Check sheet for the modelled part. Datum: model origin and axes. Units: mm. Face numbers are marked on the shaded views. A direction names the side the tool comes from. Round coordinates to 2 decimals unless told otherwise and drop trailing zeros. Order: outer loops, then holes, each group sorted by start corner. A loop starts at its lowest first (then second) coordinate and runs counter-clockwise, first axis right, second up.
```python
from build123d import *

# Parameters (mm, degrees)
CROQUIS1_R              = 10
SALIENTE_EXTRUIR1_DEPTH = 3.96875
CROQUIS3_W              = 30
CROQUIS3_H              = 7.9375
SALIENTE_EXTRUIR2_DEPTH = 30
CROQUIS4_R              = 3.175
CORTAR_EXTRUIR1_DEPTH   = 60


with BuildPart() as part:
    # Croquis1 → Saliente-Extruir1 (new, symmetric)
    with BuildSketch(Plane.XY):
        with BuildLine():
            Line((-30, -20), (30, -20))
            Line((30, -20), (30, 0))
            ThreePointArc((30, 0), (24.142135624, 14.142135624), (10, 20))
            Line((10, 20), (-10, 20))
            ThreePointArc((-10, 20), (-24.142135624, 14.142135624), (-30, 0))
            Line((-30, 0), (-30, -20))
        make_face()
        Circle(CROQUIS1_R, mode=Mode.SUBTRACT)
    extrude(amount=SALIENTE_EXTRUIR1_DEPTH, both=True)

    # Croquis3 → Saliente-Extruir2 (add, symmetric)
    with BuildSketch(Plane(origin=(0, 0, 0), x_dir=(0, 0, -1), z_dir=(1, 0, 0))):
        with Locations((-18.96875, -16.03125)):
            Rectangle(CROQUIS3_W, CROQUIS3_H)
        with Locations((18.96875, -16.03125)):
            Rectangle(CROQUIS3_W, CROQUIS3_H)
    extrude(amount=SALIENTE_EXTRUIR2_DEPTH, both=True)

    # Croquis4 → Cortar-Extruir1 (cut)
    with BuildSketch(Plane.XZ.offset(20)):
        with Locations(Location((-22, 25.96875, 0), (0, 0, 270))):
            Circle(CROQUIS4_R)
        with Locations(Location((22, 25.96875, 0), (0, 0, 270))):
            Circle(CROQUIS4_R)
        with Locations(Location((22, -25.96875, 0), (0, 0, 270))):
            Circle(CROQUIS4_R)
        with Locations(Location((-22, -25.96875, 0), (0, 0, 270))):
            Circle(CROQUIS4_R)
    extrude(amount=-CORTAR_EXTRUIR1_DEPTH, mode=Mode.SUBTRACT)


solid = part.part
```
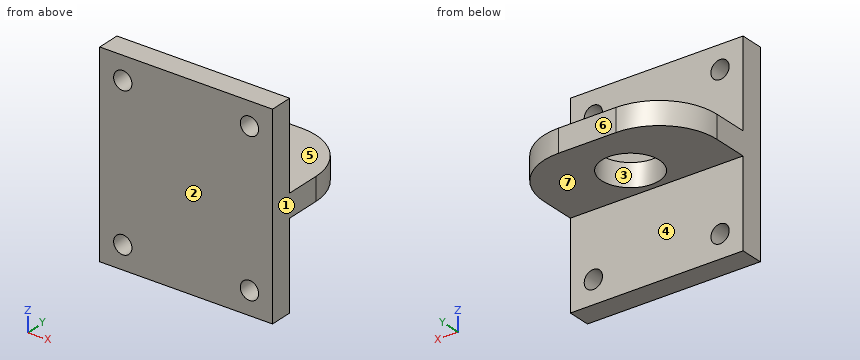
Item 1: Go/stop test with flat-tipped pins: P1, Ø8, axis at x = -10, y = 12.5, coming from the +Z side; P2, Ø15, axis at x = 2.5, z = 25.5, coming from the +Y side; P3, Ø1.5, axis at x = 11.5, y = 5.5, coming from the -Z side. Record where each tip stops, or that it passes through.
Answer:
P1: stops at z = 3.97
P2: stops at y = -12.06
P3: stops at z = -3.97
Item 2: Sectioned sample at A-A (x = -22). Record the cut outline in (y, z), and give its area (3 significant figures).
Answer:
outline: (-20, -33.97) - (-12.06, -33.97) - (-12.06, -29.14) - (-20, -29.14) - close; (-20, -22.79) - (-12.06, -22.79) - (-12.06, -3.97) - (16, -3.97) - (16, 3.97) - (-12.06, 3.97) - (-12.06, 22.79) - (-20, 22.79) - close; (-20, 29.14) - (-12.06, 29.14) - (-12.06, 33.97) - (-20, 33.97) - close
area: 661 mm2
Item 3: Sectioned sample at B-B (x = 6). Record the cut outline in (y, z).
Answer:
outline: (-20, -33.97) - (-12.06, -33.97) - (-12.06, -3.97) - (-8, -3.97) - (-8, 3.97) - (-12.06, 3.97) - (-12.06, 33.97) - (-20, 33.97) - close; (8, -3.97) - (20, -3.97) - (20, 3.97) - (8, 3.97) - close
Item 4: Access from +Z, -Z, +X, -X, +Y, -Y to the whole of each face (thin tool, end or side, straight path). Record for the marked faces 5, 6 and 7.
Answer:
face 5: +Z, +X, -X, +Y
face 6: +Z, -Z, +X, -X, +Y
face 7: -Z, +X, -X, +Y
Item 5: Scan lines: line 1 along Y through (x, z) = (0, 1.5); line 2 along Z through (x, y) = (-24, -15.5); line 3 along Z through (x, y) = (-21, -17). Record each from-to range of solid material in increasing order.
Answer:
line 1: y = -20 to -10, 10 to 20
line 2: z = -33.97 to -28.43, -23.5 to 23.5, 28.43 to 33.97
line 3: z = -33.97 to -28.98, -22.96 to 22.96, 28.98 to 33.97
Item 6: Sectioned sample at D-D (z = -10.5). Record the cut outline in (x, y), and give its area (3 significant figures).
Answer:
outline: (-30, -20) - (30, -20) - (30, -12.06) - (-30, -12.06) - close
area: 476 mm2
Item 7: Sectioned sample at C-C (y = -7.5). Record the cut outline in (x, z), and give its area (3 significant figures).
Answer:
outline: (-30, -3.97) - (-6.61, -3.97) - (-6.61, 3.97) - (-30, 3.97) - close; (6.61, -3.97) - (30, -3.97) - (30, 3.97) - (6.61, 3.97) - close
area: 371 mm2
Item 8: Release check for a two-part mould opening along Y. For the marked faces 1, 2, 3 and 4 record: released by +Y, released by -Y, zero draft, split by the parting line, or undercut.
Answer:
face 1: zero draft
face 2: released by -Y
face 3: undercut
face 4: released by +Y
